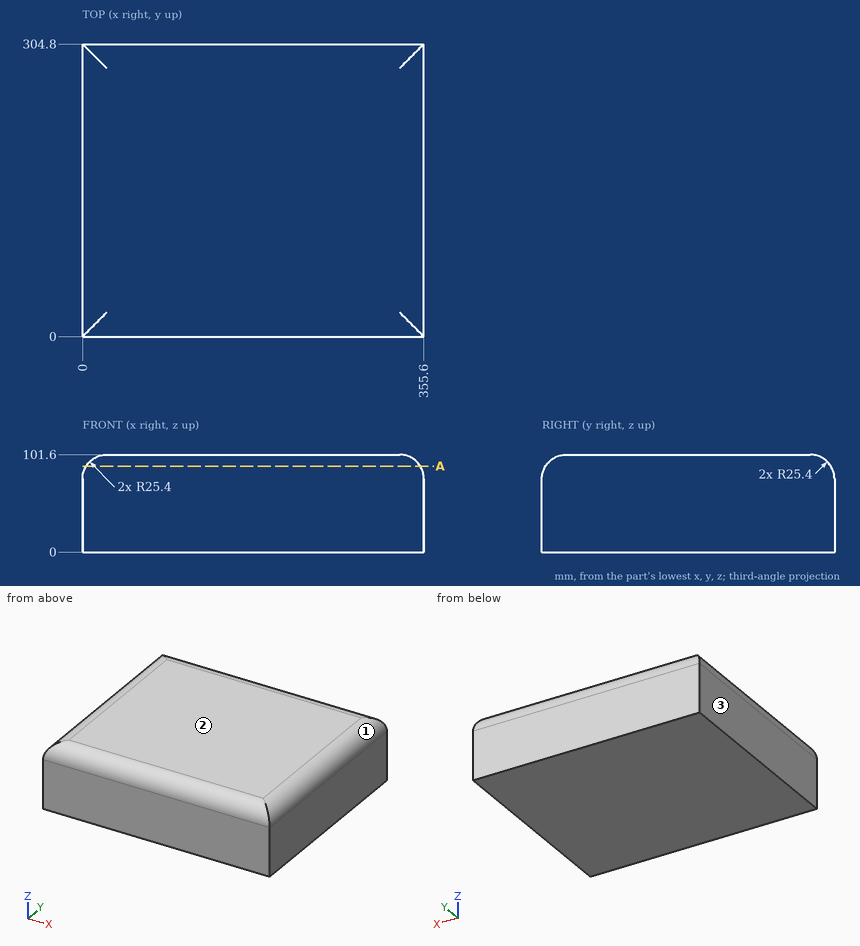
The drawing under review shows one solid part. Ordinate dimensions are in mm from its lowest x, y, z. Round coordinates to 2 decimals unless told otherwise and drop trailing zeros. Order: outer loops, then holes, each group sorted by start corner. A loop starts at its lowest first (then second) coordinate and runs counter-clockwise, first axis right, second up. Notation, with made-up numbers: (46.25, 13.5) -> (73.25, 13.5) arc R22 ccw to (73.25, 47.5) -> close; hole circle Ø8 at (33.5, -21). An arc over 180 degrees is marked (long way). Return JSON: item names as keys, results as strings.
1. Take a section at A-A (z = 89.5). Write out the cut boundary in (x, y), then the cut area to 3 significant figures.
Answer block:
{"outline": "(3.76, 3.76) -> (351.84, 3.76) -> (351.84, 301.04) -> (3.76, 301.04) -> close", "area": "103,000 mm²"}
2. For L1, parallel to Z at x = 331.5, y = 40; L2, parallel to Y at x = 165, z = 90.5; L3, parallel to Z at x = 15, y = 192, list the stretches that pass through material, from the lowest coordinate up. Write a range as [from, to].
Answer block:
{"L1": "z = [0, 101.57]", "L2": "y = [4.41, 300.39]", "L3": "z = [0, 99.37]"}
3. Insertion check: P1, Ø4, axis at y = 273, z = 83.5, coming from the -X side; P2, Ø2, axis at x = 89, y = 58.5, coming from the -Z side; P3, Ø6, axis at y = 163.5, z = 83, coming from the -X side. Each pin has a flat end and moves straight along its axis. Give the tip position at first contact, or say it passes through.
Answer block:
{"P1": "stops at x = 0.56", "P2": "stops at z = 0", "P3": "stops at x = 0.29"}
4. The part is to be moulded in two halves that separate along X. For the marked faces 1, 2 and 3, say which applies: +X half, -X half, draft (parallel to the pull), parting line (faces both ways), or undercut.
Answer block:
{"face 1": "+X half", "face 2": "draft", "face 3": "-X half"}
